from build123d import *

# Parameters (mm, degrees)
SKETCH1_R           = 2.4
BOSS_EXTRUDE1_DEPTH = 3.9
SKETCH2_R           = 3.05
CUT_EXTRUDE1_DEPTH  = 0.8
SKETCH3_R           = 3.05
CUT_EXTRUDE2_DEPTH  = 0.8


with BuildPart() as part:
    # Sketch1 → Boss-Extrude1 (new body)
    with BuildSketch(Plane(origin=(0, 0, 0), x_dir=(1, 0, 0), z_dir=(0, 1, 0))):
        with BuildLine():
            Line((-8.035, 3.65), (8.035, 3.65))
            ThreePointArc((8.035, 3.65), (11.685, 0), (8.035, -3.65))
            Line((8.035, -3.65), (-8.035, -3.65))
            ThreePointArc((-8.035, -3.65), (-11.685, 0), (-8.035, 3.65))
        make_face()
        Circle(SKETCH1_R, mode=Mode.SUBTRACT)
        Polygon((7.135, 2.4), (7.135, 0.9), (5.635, 0.9), (5.635, -0.9), (7.135, -0.9), (7.135, -2.4), (8.935, -2.4), (8.935, -0.9), (10.435, -0.9), (10.435, 0.9), (8.935, 0.9), (8.935, 2.4), align=None, mode=Mode.SUBTRACT)
        Polygon((-8.934958517, 2.400106294), (-8.934958517, 0.900106294), (-10.434958517, 0.900106294), (-10.434958517, -0.899893706), (-8.934958517, -0.899893706), (-8.934958517, -2.399893706), (-7.134958517, -2.399893706), (-7.134958517, -0.899893706), (-5.634958517, -0.899893706), (-5.634958517, 0.900106294), (-7.134958517, 0.900106294), (-7.134958517, 2.400106294), align=None, mode=Mode.SUBTRACT)
    extrude(amount=BOSS_EXTRUDE1_DEPTH)

    # Sketch2 → Cut-Extrude1 (cut)
    with BuildSketch(Plane(origin=(0, 3.9, 0), x_dir=(1, 0, 0), z_dir=(0, 1, 0))):
        Circle(SKETCH2_R)
    extrude(amount=-CUT_EXTRUDE1_DEPTH, mode=Mode.SUBTRACT)

    # Sketch3 → Cut-Extrude2 (cut)
    with BuildSketch(Plane(origin=(0, 0, 0), x_dir=(-1, 0, 0), z_dir=(0, -1, 0))):
        Circle(SKETCH3_R)
    extrude(amount=-CUT_EXTRUDE2_DEPTH, mode=Mode.SUBTRACT)


solid = part.part
Input: part model. Units: mm. Frame: model coordinates. A direction names the side the tool comes from. Coordinates: 2 decimals unless noted, no trailing zeros. Write each loop counter-clockwise with the first axis right and the second up, starting at its lowest first coordinate (ties: lowest second). Pieces come first, ordered by that corner, then holes. Notation, with made-up numbers: M -10.75,3.25 L 6.25,3.25 A22 ccw 6.25,18.25 Z; hole C -40,5 d4. An arc over 180 degrees is marked long. Answer as a JSON object with one key per item and string values. Group by question number.
(1) Mould query, pull axis X, two halves, no side actions, for faces 1 (the face through (5.635, 2, 0)), 2 (the face through (-3.047, 3.506, -0.134)), 3 (the face through (0, 2, -3.65)), 4 (the face through (11.684, 1.923, -0.08)). Classes: pulls with the +X half, pulls with the -X half, needs draft (parallel to the pull), parting line crosses it, or undercut.
(2) Section A-A on x = 0. Output: boundary loops of the cut face in (y, z).
(3) Section B-B on y = 1.7. Give the number of separate pieces and of enclosed holes in the cut face, plus the area to 3 significant figures.
(4) Set-up query: faces 5 (the face through (3, 3.9, -2)), 6 (the face through (2, 0.8, 2)), 7 (the face through (0, 2, 3.65)), 8 (the face through (-6, 2, 0.9)), 9 (the face through (-2, 3.1, 2)). Return all of +Z, -Z, +X, -X, +Y, -Y with unobstructed straight access to the full face (end or side cutting, diameter ignored); none if empty.
(5) Ray query, line 1 along X through (y, z) = (0.3, 0) (3 decimals); line 2 along Z through (x, y) = (0, 1.55); line 3 along X through (y, z) = (2.5, 1.5) (1 decimal). Return the intervals inside material, ascending. Write a range as [from, to].
(6) Contact query for flat-ended pins moving along their axis: P1, Ø0.8, axis at y = 2, z = -2, coming from the -X side; P2, Ø1.2, axis at y = 1.5, z = -1.5, coming from the -X side; P3, Ø1.6, axis at y = 3, z = -1.5, coming from the +X side. Output: stop coordinate, or through.
(7) Section C-C on z = 0. Output: boundary loops of the cut face in (x, y) (3 decimals).
Result set:
{
 "1": {"face 1": "undercut", "face 2": "undercut", "face 3": "needs draft", "face 4": "pulls with the +X half"},
 "2": {"outline": "M 0,-3.65 L 3.9,-3.65 L 3.9,-3.05 L 3.1,-3.05 L 3.1,-2.4 L 0.8,-2.4 L 0.8,-3.05 L 0,-3.05 Z; M 0,3.05 L 0.8,3.05 L 0.8,2.4 L 3.1,2.4 L 3.1,3.05 L 3.9,3.05 L 3.9,3.65 L 0,3.65 Z"},
 "3": {"separate pieces": "1", "enclosed holes": "3", "area": "113 mm2"},
 "4": {"face 5": "+Z, -Z, +X, -X, +Y", "face 6": "-Y", "face 7": "+Z, +X, -X, +Y, -Y", "face 8": "+Y, -Y", "face 9": "+Y"},
 "5": {"line 1": "x = [-11.685, -10.435], [-5.635, -3.05], [3.05, 5.635], [10.435, 11.685]", "line 2": "z = [-3.65, -2.4], [2.4, 3.65]", "line 3": "x = [-11.4, -8.9], [-7.1, -1.9], [1.9, 7.1], [8.9, 11.4]"},
 "6": {"P1": "stops at x = -11.32", "P2": "stops at x = -11.57", "P3": "stops at x = 11.62"},
 "7": {"outline": "M -11.685,0 L -10.435,0 L -10.435,3.9 L -11.685,3.9 Z; M -5.635,0 L -3.05,0 L -3.05,0.8 L -2.4,0.8 L -2.4,3.1 L -3.05,3.1 L -3.05,3.9 L -5.635,3.9 Z; M 2.4,0.8 L 3.05,0.8 L 3.05,0 L 5.635,0 L 5.635,3.9 L 3.05,3.9 L 3.05,3.1 L 2.4,3.1 Z; M 10.435,0 L 11.685,0 L 11.685,3.9 L 10.435,3.9 Z"}
}
